Answer from the drawing. Dimensions are ordinates in mm from the lowest x, y and z of the part. Give positions to 0.01 mm unless a question says otherwise; leave off trailing zeros. Order: outer loops, then holes, each group sorted by start corner. A loop starts at its lowest first (then second) coordinate and runs counter-clockwise, first axis right, second up. Notation, with made-up numbers: (49, 72) -> (90, 72) arc R31 cw to (90, 102) -> close; hole circle Ø1 at (50, 79). An arc over 180 degrees is marked (long way). Write item = value, one per line. Start each with the question number.
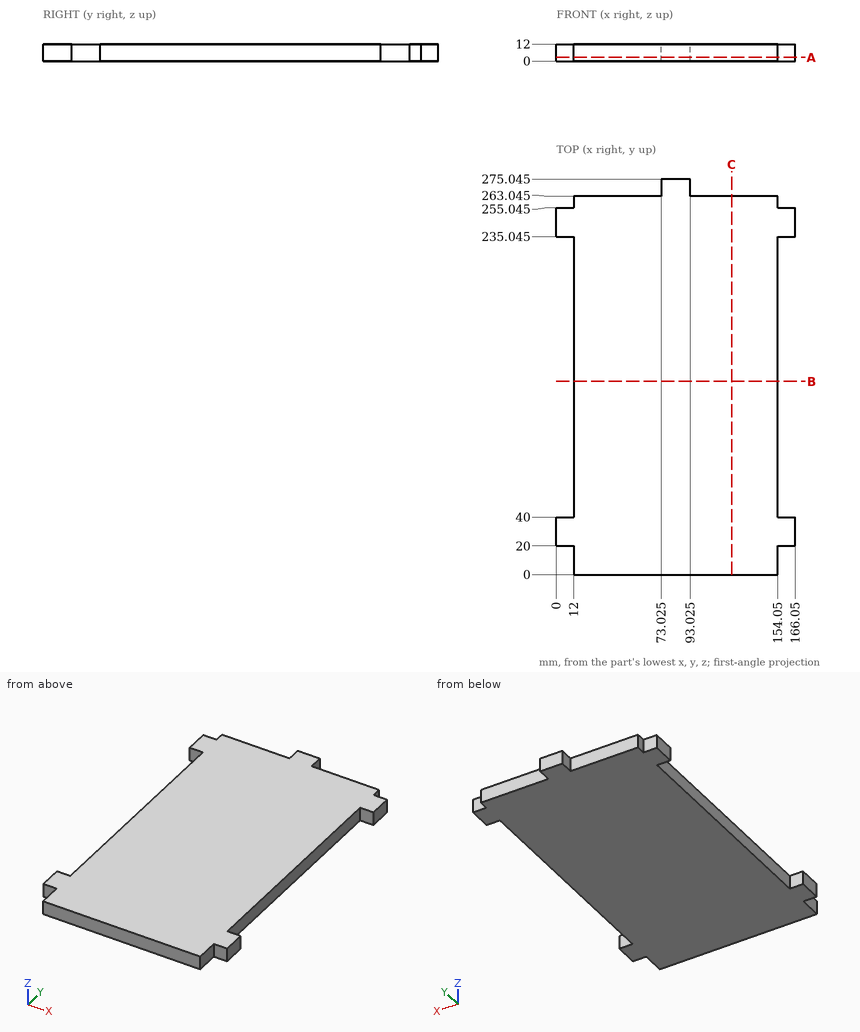
Item 1: A cutting plane is placed at C-C, the plane x = 122. Write down the section's boundary in (y, z) (3 decimals).
Item 2: A cutting plane is placed at A-A, the plane z = 2.75. Write down the section's boundary in (x, y) (3 decimals).
Item 3: A cutting plane is placed at B-B, the plane y = 134.5. Write down the section's boundary in (x, z).
Item 4: Consider L1, parallel to Y at x = 68.5, z = 7.75 (3 decimals); L2, parallel to X at y = 133, z = 5.25. Determine where each line is inside the solid, lowest interval first. Write a range as from..to.
Item 5: Flat-ended cylindrical pins translate along their axes: pin 1 (2.5 mm diameter, centred on y = 259.5, z = 3.5, fed in from -X); pin 2 (3 mm diameter, centred on x = 35.5, z = 8.5, fed in from -Y); pin 3 (1.5 mm diameter, centred on y = 103, z = 10.5, fed in from +X); pin 4 (6 mm diameter, centred on x = 5, z = 5.5, fed in from -Y). Find the tip coordinate at first contact, or state that the pin passes through.
Check values:
q1.outline = (0, 0) -> (263.045, 0) -> (263.045, 12) -> (0, 12) -> close
q2.outline = (0, 20) -> (12, 20) -> (12, 0) -> (154.05, 0) -> (154.05, 20) -> (166.05, 20) -> (166.05, 40) -> (154.05, 40) -> (154.05, 235.045) -> (166.05, 235.045) -> (166.05, 255.045) -> (154.05, 255.045) -> (154.05, 263.045) -> (93.025, 263.045) -> (93.025, 275.045) -> (73.025, 275.045) -> (73.025, 263.045) -> (12, 263.045) -> (12, 255.045) -> (0, 255.045) -> (0, 235.045) -> (12, 235.045) -> (12, 40) -> (0, 40) -> close
q3.outline = (12, 0) -> (154.05, 0) -> (154.05, 12) -> (12, 12) -> close
q4.L1 = 0..263.045
q4.L2 = 12..154.05
q5.pin_1 = 12
q5.pin_2 = 0
q5.pin_3 = 154.05
q5.pin_4 = 20
